```python
from build123d import *

# Parameters (mm, degrees)
SKETCH1_R           = 1.5
BOSS_EXTRUDE1_DEPTH = 1.7
FILLET1_R           = 15
FILLET2_R           = 2


with BuildPart() as part:
    # Sketch1 → Boss-Extrude1 (new body)
    with BuildSketch(Plane.XY):
        with BuildLine():
            ThreePointArc((-11.978690547, -106.87499991), (9.060608653, -104.164298748), (6.349906949, -83.124999619))
            ThreePointArc((6.349906949, -83.124999619), (-22.020584843, -49.648176002), (-34.231800328, -7.5))
            Line((-34.231800328, -7.5), (-9.5, -7.5))
            Line((-9.5, -7.5), (-2, 0))
            Line((-2, 0), (-9.5, 7.5))
            Line((-9.5, 7.5), (-34.231800328, 7.5))
            ThreePointArc((-34.231800328, 7.5), (-22.020584884, 49.648175925), (6.349906811, 83.124999512))
            ThreePointArc((6.349906811, 83.124999512), (9.060608694, 104.164298694), (-11.978690577, 106.874999887))
            ThreePointArc((-11.978690577, 106.874999887), (-64.5, -1.9e-08), (-11.978690547, -106.87499991))
        make_face()
        with Locations((-14.5, 0)):
            Circle(SKETCH1_R, mode=Mode.SUBTRACT)
    extrude(amount=BOSS_EXTRUDE1_DEPTH)

    # Fillet1
    fillet1_edges = [part.edges().sort_by_distance(p)[0] for p in [
        (-34.231800328, -7.5, 0.85),
        (-34.231800328, 7.5, 0.85),
    ]]
    fillet(fillet1_edges, radius=FILLET1_R)

    # Fillet2
    fillet2_edges = [part.edges().sort_by_distance(p)[0] for p in [
        (-9.5, 7.5, 0.85),
        (-2, 0, 0.85),
        (-9.5, -7.5, 0.85),
    ]]
    fillet(fillet2_edges, radius=FILLET2_R)


solid = part.part
```
For this review, take the finished solid that the model builds, in its own axes (mm). A direction names the side the tool comes from. Round coordinates to 2 decimals unless told otherwise and drop trailing zeros. Write each loop counter-clockwise with the first axis right and the second up, starting at its lowest first coordinate (ties: lowest second). Pieces come first, ordered by that corner, then holes. Notation, with made-up numbers: (12, 3.25) - (18, 3.25) arc R24 cw to (18, 41.25) - close; hole circle Ø1 at (15, 6.25). An arc over 180 degrees is marked (long way). Answer as a JSON object with one key per item and string values.
1. For pin 1 Ø1 at (y, z) = (6, 1) entering from +X, flat-tipped, find the tip position at first contact; note if it passes through.
Response values:
{"pin 1": "stops at x = -7.5"}
2. We need section A-A on z = 0.6. Give the boundary of the cut face in (x, y) (3 decimals).
Response values:
{"outline": "(-31.166, -26.25) arc R15 cw to (-16.642, -7.5) - (-10.328, -7.5) arc R2 ccw to (-8.914, -6.914) - (-3.414, -1.414) arc R2 ccw to (-3.414, 1.414) - (-8.914, 6.914) arc R2 ccw to (-10.328, 7.5) - (-16.642, 7.5) arc R15 cw to (-31.166, 26.25) arc R105 cw to (6.35, 83.125) arc R15 ccw to (-11.979, 106.875) arc R135 ccw to (-11.979, -106.875) arc R15 ccw to (6.35, -83.125) arc R105 cw to start; hole circle Ø3 at (-14.5, 0)"}
3. Tool access review of faces 4 (the face through (-17.416, 57.409, 0.838)), 5 (the face through (8.86, -104.42, 0.84)): name each direction out of +Z, -Z, +X, -X, +Y, -Y from which nothing blocks a thin tool from reaching the whole face with its end or side.
Response values:
{"face 4": "+Z, -Z, +X", "face 5": "+Z, -Z"}
4. Draft analysis for pull direction Y (two halves, no side actions). For faces 1 (the face through (-64.49, 1.73, 0.84)), 2 (the face through (-27, 2, 0)), 3 (the face through (-6, 4, 1)), state which applies: +Y half, -Y half, draft (parallel to the pull), parting line (faces both ways), or undercut.
Response values:
{"face 1": "parting line", "face 2": "draft", "face 3": "undercut"}
5. We need section C-C on y = 59.5. Give the boundary of the cut face in (x, z), then the cut area to 3 significant figures.
Response values:
{"outline": "(-50.68, 0) - (-16.01, 0) - (-16.01, 1.7) - (-50.68, 1.7) - close", "area": "58.9 mm2"}
6. We need section B-B on x = -54. Give the boundary of the cut face in (y, z), then the cut area to 3 significant figures.
Response values:
{"outline": "(-52.2, 0) - (52.2, 0) - (52.2, 1.7) - (-52.2, 1.7) - close", "area": "177 mm2"}
7. To check wall thickness, follow line 1 along Y through (x, z) = (-14.5, 1.35); line 2 along Y through (x, z) = (-22.5, 1.35); line 3 along Y through (x, z) = (-19.5, 1.25). State the ranges of each line that lie inside material, in increasing order.
Response values:
{"line 1": "y = -104.88 to -61.64, -7.5 to -1.5, 1.5 to 7.5, 61.64 to 104.88", "line 2": "y = -97.86 to -48.74, -8.69 to 8.69, 48.74 to 97.86", "line 3": "y = -100.62 to -54.08, -7.77 to 7.77, 54.08 to 100.62"}
